```python
from build123d import *

# Parameters (mm, degrees)
SKETCH1_W                                           = 76.2
SKETCH1_H                                           = 25.4
BOSS_EXTRUDE1_DEPTH                                 = 31.75
CUT_EXTRUDE1_REACH                                  = 85.521
SKETCH2_W                                           = 15.24
SKETCH2_H                                           = 19.05
SKETCH3_R                                           = 3.175
CUT_EXTRUDE2_DEPTH                                  = 56.72102386
LPATTERN1_COUNT                                     = 5
LPATTERN1_PITCH                                     = 12.7
CBORE_FOR_6_BINDING_HEAD_MACHINE_SCREW1_D           = 3.7973
CBORE_FOR_6_BINDING_HEAD_MACHINE_SCREW1_CBORE_D     = 7.9375
CBORE_FOR_6_BINDING_HEAD_MACHINE_SCREW1_CBORE_DEPTH = 2.2098
FILLET2_R                                           = 7.62
CUT_EXTRUDE3_REACH                                  = 57.721
SKETCH7_W                                           = 12.7
SKETCH7_H                                           = 6.35
SKETCH7_W_2                                         = 25.4
FILLET5_R                                           = 6.35
FILLET6_R                                           = 2.54


# Some blends are built 0.0001 mm under size
with BuildPart() as part:
    # Sketch1 → Boss-Extrude1 (new body)
    with BuildSketch(Plane(origin=(0, 0, 0), x_dir=(1, 0, 0), z_dir=(0, 1, 0))):
        Rectangle(SKETCH1_W, SKETCH1_H)
    extrude(amount=BOSS_EXTRUDE1_DEPTH)

    # Sketch2 → Cut-Extrude1 (cut, up to next)
    with BuildSketch(Plane(origin=(38.1, 0, 0), x_dir=(0, 0, -1), z_dir=(1, 0, 0)), mode=Mode.PRIVATE) as cut_extrude1_sk1:
        with Locations((0, 22.225)):
            Rectangle(SKETCH2_W, SKETCH2_H)
    cut_extrude1_tool1 = extrude(cut_extrude1_sk1.sketch, amount=-CUT_EXTRUDE1_REACH, mode=Mode.PRIVATE) & part.part
    add(cut_extrude1_tool1.solids().sort_by_distance((38.1, 22.225, 0))[0], mode=Mode.SUBTRACT)

    # Sketch3 → Cut-Extrude2 (cut, through all)
    with BuildSketch(Plane.XY.offset(12.7)):
        with Locations((-25.4, 25.4)):
            Circle(SKETCH3_R)
    cut_extrude2 = extrude(amount=-CUT_EXTRUDE2_DEPTH, mode=Mode.SUBTRACT)

    # LPattern1: Cut-Extrude2 ×5
    with Locations(*[(i * LPATTERN1_PITCH, 0, 0) for i in range(1, LPATTERN1_COUNT)]):
        add(cut_extrude2, mode=Mode.SUBTRACT)

    # CBORE for #6 Binding Head Machine Screw1 (through all)
    with Locations(Plane(origin=(0, 12.7, 0), x_dir=(1, 0, 0), z_dir=(0, 1, 0))):
        with Locations((-19.05, 0), (19.05, 0)):
            CounterBoreHole(CBORE_FOR_6_BINDING_HEAD_MACHINE_SCREW1_D / 2, CBORE_FOR_6_BINDING_HEAD_MACHINE_SCREW1_CBORE_D / 2, CBORE_FOR_6_BINDING_HEAD_MACHINE_SCREW1_CBORE_DEPTH)

    # Fillet2
    # the kernel refuses this fillet: 7.62 mm, written as the material it adds along each edge
    with BuildSketch(Plane(origin=(38.1, 12.7, -7.62), x_dir=(0, 1, 0), z_dir=(-1, 0, 0))) as fillet2_piece_1_section:
        with BuildLine():
            CenterArc((FILLET2_R, -FILLET2_R), FILLET2_R, 90, 90)
            Line((0, -FILLET2_R), (0, 0))
            Line((0, 0), (FILLET2_R, 0))
        make_face()
    fillet2_piece_1 = extrude(amount=76.2, mode=Mode.PRIVATE)
    fillet2_piece_1 = fillet2_piece_1 - Plane(origin=(-19.05, 14.454782772, 0), x_dir=(1, 0, 0), z_dir=(0, 1, 0)) * Cylinder(3.96875, 183, mode=Mode.PRIVATE)
    fillet2_piece_1 = fillet2_piece_1 - Plane(origin=(19.05, 14.454782772, 0), x_dir=(1, 0, 0), z_dir=(0, 1, 0)) * Cylinder(3.96875, 183, mode=Mode.PRIVATE)
    add(fillet2_piece_1)
    with BuildSketch(Plane(origin=(38.1, 12.7, 7.62), x_dir=(0, 0, -1), z_dir=(-1, 0, 0))) as fillet2_piece_2_section:
        with BuildLine():
            CenterArc((FILLET2_R, -FILLET2_R), FILLET2_R, 90, 90)
            Line((0, -FILLET2_R), (0, 0))
            Line((0, 0), (FILLET2_R, 0))
        make_face()
    fillet2_piece_2 = extrude(amount=76.2, mode=Mode.PRIVATE)
    fillet2_piece_2 = fillet2_piece_2 - Plane(origin=(-19.05, 14.454782936, 0), x_dir=(1, 0, 0), z_dir=(0, 1, 0)) * Cylinder(3.96875, 183, mode=Mode.PRIVATE)
    fillet2_piece_2 = fillet2_piece_2 - Plane(origin=(19.05, 14.454782936, 0), x_dir=(1, 0, 0), z_dir=(0, 1, 0)) * Cylinder(3.96875, 183, mode=Mode.PRIVATE)
    add(fillet2_piece_2)

    # Sketch7 → Cut-Extrude3 (cut, up to next)
    with BuildSketch(Plane.XY.offset(12.7), mode=Mode.PRIVATE) as cut_extrude3_sk1:
        with Locations((-31.75, 3.175)):
            Rectangle(SKETCH7_W, SKETCH7_H)
    cut_extrude3_tool1 = extrude(cut_extrude3_sk1.sketch, amount=-CUT_EXTRUDE3_REACH, mode=Mode.PRIVATE) & part.part
    # Sketch7 → Cut-Extrude3 (cut, up to next)
    with BuildSketch(Plane.XY.offset(12.7), mode=Mode.PRIVATE) as cut_extrude3_sk2:
        with Locations((31.75, 3.175)):
            Rectangle(SKETCH7_W, SKETCH7_H)
    cut_extrude3_tool2 = extrude(cut_extrude3_sk2.sketch, amount=-CUT_EXTRUDE3_REACH, mode=Mode.PRIVATE) & part.part
    # Sketch7 → Cut-Extrude3 (cut, up to next)
    with BuildSketch(Plane.XY.offset(12.7), mode=Mode.PRIVATE) as cut_extrude3_sk3:
        with Locations((0, 3.175)):
            Rectangle(SKETCH7_W_2, SKETCH7_H)
    cut_extrude3_tool3 = extrude(cut_extrude3_sk3.sketch, amount=-CUT_EXTRUDE3_REACH, mode=Mode.PRIVATE) & part.part
    add(cut_extrude3_tool1.solids().sort_by_distance((-31.75, 3.175, 12.7))[0], mode=Mode.SUBTRACT)
    add(cut_extrude3_tool2.solids().sort_by_distance((31.75, 3.175, 12.7))[0], mode=Mode.SUBTRACT)
    add(cut_extrude3_tool3.solids().sort_by_distance((0, 3.175, 12.7))[0], mode=Mode.SUBTRACT)

    # Fillet5
    fillet5_edges = [part.edges().sort_by_distance(p)[0] for p in [
        (-25.4, 6.35, 0),
        (-12.7, 6.35, 0),
        (12.7, 6.35, 0),
        (25.4, 6.35, 0),
    ]]
    fillet(fillet5_edges, radius=FILLET5_R - 0.0001)  # a hair under: the kernel refuses the full size

    # Fillet6
    fillet6_edges = [part.edges().sort_by_distance(p)[0] for p in [
        (-38.1, 19.05, -12.7),
        (38.1, 19.05, -12.7),
        (38.1, 19.05, 12.7),
        (-38.1, 19.05, 12.7),
    ]]
    fillet(fillet6_edges, radius=FILLET6_R)


solid = part.part
```
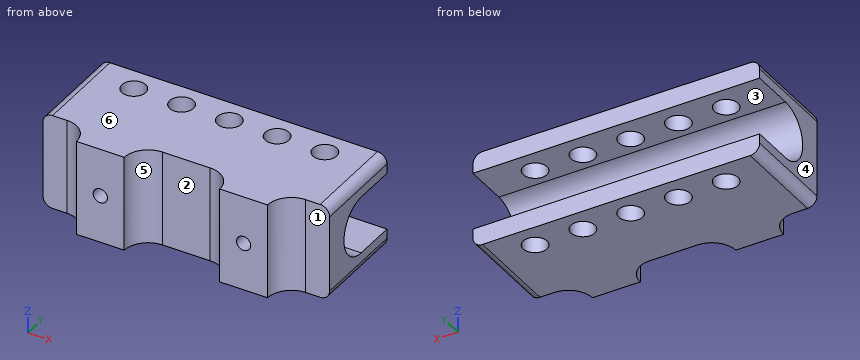
Build history of the part. All positions in model axes, mm. Face numbers are marked on the shaded views. A direction names the side the tool comes from. Coordinates: 2 decimals unless noted, no trailing zeros. Write each loop counter-clockwise with the first axis right and the second up, starting at its lowest first coordinate (ties: lowest second). Pieces come first, ordered by that corner, then holes.
1. 3-axis set-ups, long thin cutter, end or side, ignore diameter. For the marked faces 1, 2 and 3: which of +Z, -Z, +X, -X, +Y, -Y reach the whole face in a straight line?
Answer block:
face 1: +Z, -Z, +X, -Y
face 2: +Z, -Z, -Y
face 3: +X, -X, +Y
2. Band-saw the part on B-B, the plane x = 0. Give the cut face in (y, z) (3 decimals).
Answer block:
outline: (6.35, -12.7) - (22.225, -12.7) - (22.225, -7.62) - (20.32, -7.62) arc R7.62 cw to (20.32, 7.62) - (22.225, 7.62) - (22.225, 12.7) - (6.35, 12.7) - close; (28.575, -12.7) - (31.75, -12.7) - (31.75, -7.62) - (28.575, -7.62) - close; (28.575, 7.62) - (31.75, 7.62) - (31.75, 12.7) - (28.575, 12.7) - close
3. Drop flat-ended pins along their axis: pin 1 (4 mm diameter, centred on x = 1.5, z = 6, fed in from -Y); pin 2 (4.5 mm diameter, centred on x = 19.05, z = 0, fed in from +Y); pin 3 (1.9 mm diameter, centred on x = 35.5, z = 6.5, fed in from -Y). Give the stop position or say it passes through.
Answer block:
pin 1: stops at y = 6.35
pin 2: stops at y = 10.49
pin 3: stops at y = 6.35
4. Band-saw the part on C-C, the plane y = 3. Give the cut face in (x, z).
Answer block:
outline: (-26.15, -12.7) - (-11.95, -12.7) - (-11.95, 12.7) - (-26.15, 12.7) - close; (11.95, -12.7) - (26.15, -12.7) - (26.15, 12.7) - (11.95, 12.7) - close; hole circle Ø3.8 at (-19.05, 0); hole circle Ø3.8 at (19.05, 0)
5. Drill centre lines: probe 1 along Z at (x, y) = (26, 21.5); probe 2 along Y at (x, z) = (0, -8.25) (3 decimals); probe 3 along X at (y, z) = (24, 11.5). Where is each one in solid material? Low to high.
Answer block:
probe 1: z = -12.7 to -7.62, 7.62 to 12.7
probe 2: y = 6.35 to 22.225, 28.575 to 31.75
probe 3: x = -37.72 to -28.25, -22.55 to -15.55, -9.85 to -2.85, 2.85 to 9.85, 15.55 to 22.55, 28.25 to 37.72
6. Band-saw the part on A-A, the plane y = 21.5. Give the cut face in (x, z), and give its area (3 significant figures).
Answer block:
outline: (-38.1, -10.16) arc R2.54 ccw to (-35.56, -12.7) - (35.56, -12.7) arc R2.54 ccw to (38.1, -10.16) - (38.1, -7.62) - (-38.1, -7.62) - close; (-38.1, 7.62) - (38.1, 7.62) - (38.1, 10.16) arc R2.54 ccw to (35.56, 12.7) - (-35.56, 12.7) arc R2.54 ccw to (-38.1, 10.16) - close
area: 769 mm2
7. Pull direction X, two halves, no side cores. Call the marked faces 4, 5 and 6: released by +X, released by -X, zero draft, split by the parting line, or undercut.
Answer block:
face 4: released by -X
face 5: undercut
face 6: zero draft
